Verification items for the finished model (mm, model axes). A direction names the side the tool comes from. Give positions to 0.01 mm unless a question says otherwise; leave off trailing zeros. Order: outer loops, then holes, each group sorted by start corner. A loop starts at its lowest first (then second) coordinate and runs counter-clockwise, first axis right, second up. Notation, with made-up numbers: (49, 24.25) - (90, 24.25) arc R14 ccw to (90, 40.25) - close; hole circle Ø5 at (-4, -7). An arc over 180 degrees is marked (long way). Answer as a JSON object with one key per item and string values. Group by question number.
(1) Section check B-B (x = -139). Record the boundary of the cut face in (y, z) (3 decimals).
(2) Thickness scan on line 1 (X direction, y = 16, z = 261) (3 decimals); line 2 (Y direction, x = 361, z = 268.5) (3 decimals). Record the ranges inside material, lowest first.
(3) Access from +Z, -Z, +X, -X, +Y, -Y to the whole of each face (thin tool, end or side, straight path). Record for faces 4 (the face through (475, -263.525, 270)), 5 (the face through (946, -231.775, 270)).
(4) Section check C-C (y = 24.5). Record the boundary of the cut face in (x, z) (3 decimals).
(5) Mould release check, pull along X, two halves, no side actions. Record for faces 1 (the face through (-479.425, 4, 270)), 2 (the face through (-6, 231.775, 270)), 3 (the face through (503, 263.525, 270)): +X half, -X half, draft (parallel to the pull), parting line (faces both ways), or undercut.
(6) Section check A-A (z = 278.5). Record the boundary of the cut face in (x, y) (3 decimals).
```python
from build123d import *

# Parameters (mm, degrees)
F1_W     = 895.35
F1_H     = 463.55
F1_W_2   = 946.15
F2_DEPTH = 31.75


with BuildPart() as f2:
    # F1 (on offset) → F2 (new body)
    with BuildSketch(Plane.XY.offset(254)):
        Polygon((1457.325, 263.525), (479.425, 263.525), (-479.425, 263.525), (-479.425, -263.525), (479.425, -263.525), (1457.325, -263.525), align=None)
        Rectangle(F1_W, F1_H, mode=Mode.SUBTRACT)
        with Locations((952.5, 0)):
            Rectangle(F1_W_2, F1_H, mode=Mode.SUBTRACT)
    extrude(amount=F2_DEPTH)


solid = f2.part
```
Solutions:
{
 "1": {"outline": "(-263.525, 254) - (-231.775, 254) - (-231.775, 285.75) - (-263.525, 285.75) - close; (231.775, 254) - (263.525, 254) - (263.525, 285.75) - (231.775, 285.75) - close"},
 "2": {"line 1": "x = -479.425 to -447.675, 447.675 to 479.425, 1425.575 to 1457.325", "line 2": "y = -263.525 to -231.775, 231.775 to 263.525"},
 "3": {"face 4": "+Z, -Z, +X, -X, -Y", "face 5": "+Z, -Z"},
 "4": {"outline": "(-479.425, 254) - (-447.675, 254) - (-447.675, 285.75) - (-479.425, 285.75) - close; (447.675, 254) - (479.425, 254) - (479.425, 285.75) - (447.675, 285.75) - close; (1425.575, 254) - (1457.325, 254) - (1457.325, 285.75) - (1425.575, 285.75) - close"},
 "5": {"face 1": "-X half", "face 2": "undercut", "face 3": "draft"},
 "6": {"outline": "(-479.425, -263.525) - (1457.325, -263.525) - (1457.325, 263.525) - (-479.425, 263.525) - close; hole (-447.675, -231.775) - (447.675, -231.775) - (447.675, 231.775) - (-447.675, 231.775) - close; hole (479.425, -231.775) - (1425.575, -231.775) - (1425.575, 231.775) - (479.425, 231.775) - close"}
}
